Autodesk Inventor part; units mm, degrees
ref_plane "YZ Plane" through (0, 0, 0) normal (1, 0, 0) x (0, 1, 0)
ref_plane "XZ Plane" through (0, 0, 0) normal (0, 1, 0) x (-1, 0, 0)
ref_plane "XY Plane" through (0, 0, 0) normal (0, 0, 1) x (1, 0, 0)
sketch "Sketch1" plane through (0, 0, 0) normal (0, 0, 1) x (1, 0, 0)
  line L0 (0, 0) -> (42.4, 0)
  line L1 (42.4, 0) -> (42.4, 24)
  line L2 (42.4, 24) -> (0, 24)
  line L3 (0, 24) -> (0, 0)
  circle A0 centre (9.2, 20) radius 2.1
  circle A1 centre (33.2, 20) radius 2.1
  circle A2 centre (33.2, 4) radius 2.1
  circle A3 centre (9.2, 4) radius 2.1
  dimension "d0" = 24
  dimension "d1" = 42.4
  dimension "d2" = 4.2
  dimension "d3" = 9.2
  dimension "d4" = 9.2
  dimension "d5" = 9.2
  dimension "d6" = 9.2
  dimension "d7" = 4
  dimension "d8" = 4
  dimension "d9" = 4
  dimension "d10" = 4
extrude "Extrusion1" add sketch "Sketch1" along normal blind 13.5
sketch "Sketch2" plane through (0, 0, 0) normal (0, -1, 0) x (1, 0, 0)
  line L0 (42.4, 13.5) -> (0, 13.5)
  line L1 (0, 0) -> (0, 13.5)
  circle A0 centre (21.2, 15) radius 7.5
  dimension "d13" = 15
  dimension "d14" = 21.2
  dimension "d15" = 1.5
extrude "Extrusion2" cut sketch "Sketch2" against normal through all
fillet "Fillet1" radius 3 3 edges at (42.4, 0, 6.75) (0, 0, 6.75) (21.2, 0, 0)
sketch "Sketch3" plane through (0, 0, 0) normal (0, 0, -1) x (-1, 0, 0)
  arc A0 (-31.3534, 3) -> (-35.0466, 3) centre (-33.2, 4) ccw
  arc A1 (-7.3534, 3) -> (-11.0466, 3) centre (-9.2, 4) ccw
  circle A2 centre (-33.2, 20) radius 2.1
  circle A3 centre (-9.2, 20) radius 2.1
  circle A4 centre (-33.2, 20) radius 4.25
  circle A5 centre (-9.2, 20) radius 4.25
  circle A6 centre (-9.2, 4) radius 4.25
  circle A7 centre (-33.2, 4) radius 4.25
  point P0 (0, 0)
  dimension "d20" = 8.5
extrude "Extrusion3" cut sketch "Sketch3" against normal blind 4
sketch "Sketch4" plane through (21.2, 0, 15) normal (0, -1, 0) x (1, 0, 0)
  line L0 (-26.3081, 1.9971) -> (24.247, 1.9971)
  line L1 (24.247, 1.9971) -> (24.247, -18.7305)
  line L2 (24.247, -18.7305) -> (-26.3081, -18.7305)
  line L3 (-26.3081, -18.7305) -> (-26.3081, 1.9971)
  point P0 (-21.2, -15)
extrude "Extrusion4" [suppressed]
fillet "Fillet3" radius 3 2 edges at (42.4, 13.5, 0) (0, 13.5, 0)
fillet "Fillet4" radius 1 7 edges at (41.5213, 24, 0.8787) (37.0181, 24, 0) (42.4, 24, 8.25) (21.2, 24, 0) (0.8787, 24, 0.8787) (0, 24, 8.25) (5.3819, 24, 0)
properties part number "Z move plate"
Build history of the part. All positions in model axes, mm. A direction names the side the tool comes from. Coordinates: 2 decimals unless noted, no trailing zeros. Order: outer loops, then holes, each group sorted by start corner. A loop starts at its lowest first (then second) coordinate and runs counter-clockwise, first axis right, second up. Notation, with made-up numbers: M 59,75 L 64,75 A28 cw 64,103 Z; hole C -7,8.25 d3. An arc over 180 degrees is marked long. One line per question, with ' | ' between items. Start each with the question number.
Q1. Saw through at D-D (x = 27). List the corners of the cut face in (y, z) (3 decimals).
Q2. Probe L1, parallel to Y at x = 33.2, z = 9.25; L2, parallel to X at y = 4, z = 10.5; L3, parallel to X at y = 3, z = 3. List the from-to ranges inside material, lowest first. Write a range as from..to.
Q3. Two-plate mould, pull along Y, no slides. Class faces 3 (the face through (37.514, 0.562, 1.252)), 4 (the face through (4.819, 23.715, 0.301)), 5 (the face through (9.034, 8.247, 1.972)): +Y half, -Y half, draft (parallel to the pull), parting line (faces both ways), or undercut.
Q4. Flat gauge pins, fed straight in: pin 1 Ø8 at (x, z) = (24.5, 2) entering from -Y; pin 2 Ø2.5 at (x, y) = (9, 3) entering from -Z; pin 3 Ø3 at (x, y) = (24.5, 5.5) entering from +Z; pin 4 Ø1.5 at (x, y) = (18.5, 2.5) entering from +Z. Where does each tip first touch, or does it go through?
Q5. Saw through at C-C (y = 9). List the corners of the cut face in (x, z).
Q6. 3-axis set-ups, long thin cutter, end or side, ignore diameter. For faces 1 (the face through (21, 13, 0)), 2 (the face through (7, 5, 4)): which of +Z, -Z, +X, -X, +Y, -Y reach the whole face in a straight line?
Q7. Saw through at A-A (x = 9.2). List the corners of the cut face in (y, z).
Q8. Saw through at B-B (y = 4). List the corners of the cut face in (x, z), then the cut area to 3 significant figures.
Check values:
1) outline: M 0,3 A3 ccw 3,0 L 23,0 A1 ccw 24,1 L 24,10.245 L 0,10.245 Z
2) L1: y = 0..1.9, 6.1..17.9, 22.1..24 | L2: x = 0..7.1, 11.3..15.2, 27.2..31.1, 35.3..42.4 | L3: x = 0..5.07, 13.33..29.07, 37.33..42.4
3) face 3: -Y half | face 4: +Y half | face 5: undercut
4) pin 1: stops at y = 0 | pin 2: stops at z = 4 | pin 3: stops at z = 9.24 | pin 4: stops at z = 8.34
5) outline: M 0,3 A3 ccw 3,0 L 39.4,0 A3 ccw 42.4,3 L 42.4,13.5 L 28.55,13.5 A7.5 cw 13.85,13.5 L 0,13.5 Z
6) face 1: -Z, +X, -X, +Y, -Y | face 2: -Z
7) outline: M 0,4 L 1.9,4 L 1.9,13.5 L 0,13.5 Z; M 6.1,4 L 8.25,4 L 8.25,0 L 15.75,0 L 15.75,4 L 17.9,4 L 17.9,13.5 L 6.1,13.5 Z; M 22.1,4 L 24,4 L 24,13.5 L 22.1,13.5 Z
8) outline: M 0,3 A3 ccw 3,0 L 4.95,0 L 4.95,4 L 7.1,4 L 7.1,13.5 L 0,13.5 Z; M 11.3,4 L 13.45,4 L 13.45,0 L 28.95,0 L 28.95,4 L 31.1,4 L 31.1,13.5 L 28.55,13.5 A7.5 cw 13.85,13.5 L 11.3,13.5 Z; M 35.3,4 L 37.45,4 L 37.45,0 L 39.4,0 A3 ccw 42.4,3 L 42.4,13.5 L 35.3,13.5 Z | area: 355 mm2
